Verification items for this drawing (mm, ordinates from the low corner). A direction names the side the tool comes from. Round coordinates to 2 decimals unless told otherwise and drop trailing zeros. Loops run counter-clockwise (first coordinate to the right, second up) from the corner with the lowest first, then second, coordinate; pieces in that order, holes last. Notation, with made-up numbers: (88, -15.5) - (125, -15.5) arc R27 cw to (125, 18.5) - close; hole circle Ø1 at (-23, -28). An arc over 180 degrees is marked (long way). Put each result on its own line as item: value.
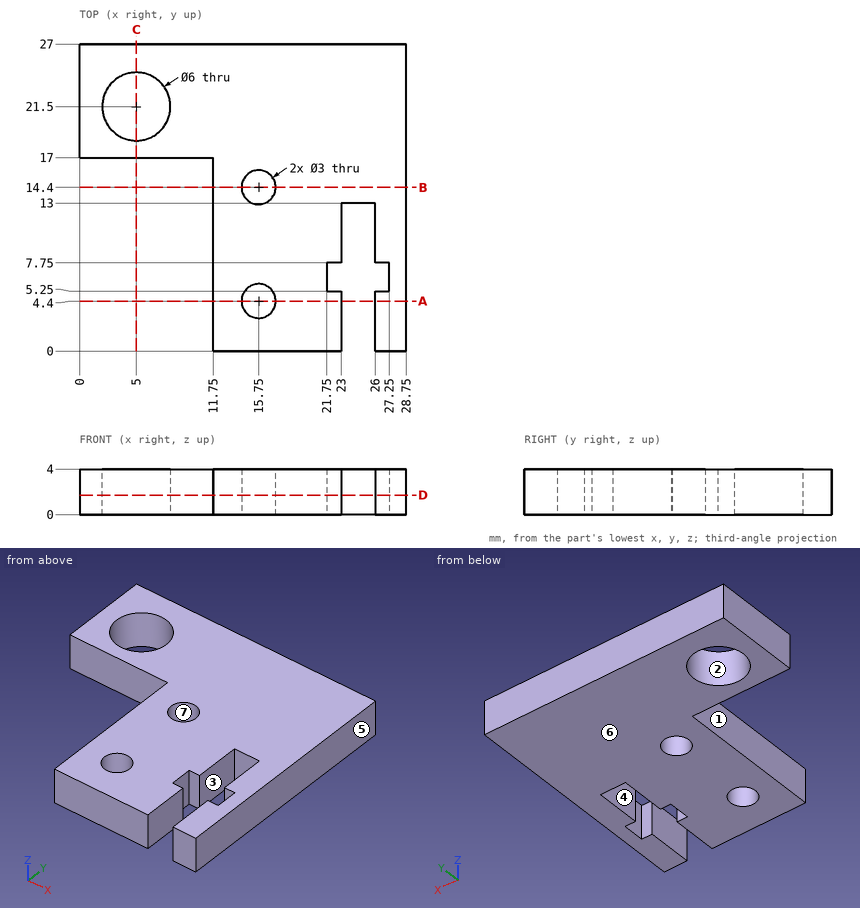
Item 1: Thickness scan on line 1 (Y direction, x = 15.75, z = 1.25); line 2 (X direction, y = 6.25, z = 3.8); line 3 (Y direction, x = 5, z = 1.95). Record the ranges inside material, lowest first. Write a range as from..to.
Filled sheet:
line 1: 0..2.9, 5.9..12.9, 15.9..27
line 2: 11.75..21.75, 27.25..28.75
line 3: 17..18.5, 24.5..27
Item 2: Go/stop test with flat-tipped pins: pin 1 (0.9 mm diameter, centred on x = 24.5, z = 1.5, fed in from -Y); pin 2 (1.2 mm diameter, centred on y = 11, z = 1.5, fed in from -X); pin 3 (1.2 mm diameter, centred on x = 7, z = 2, fed in from -Y). Record where each tip stops, or that it passes through.
Filled sheet:
pin 1: y = 13
pin 2: x = 11.75
pin 3: y = 17
Item 3: Section check D-D on z = 1.7. Enter the section's corners in (x, y), then the cut area to 3 significant figures.
Filled sheet:
outline: (0, 17) - (11.75, 17) - (11.75, 0) - (23, 0) - (23, 5.25) - (21.75, 5.25) - (21.75, 7.75) - (23, 7.75) - (23, 13) - (26, 13) - (26, 7.75) - (27.25, 7.75) - (27.25, 5.25) - (26, 5.25) - (26, 0) - (28.75, 0) - (28.75, 27) - (0, 27) - close; hole circle Ø6 at (5, 21.5); hole circle Ø3 at (15.75, 4.4); hole circle Ø3 at (15.75, 14.4)
area: 489 mm²
Item 4: Tool access check on the marked faces 1, 2 and 3. Record the directions out of +Z, -Z, +X, -X, +Y, -Y that give a thin tool (end or side, any length) a straight path to the whole face; none if there is none.
Filled sheet:
face 1: +Z, -Z, -X, -Y
face 2: +Z, -Z
face 3: +Z, -Z, -Y
Item 5: Section check C-C on x = 5. Enter the section's corners in (y, z), then the cut area to 3 significant figures.
Filled sheet:
outline: (17, 0) - (18.5, 0) - (18.5, 4) - (17, 4) - close; (24.5, 0) - (27, 0) - (27, 4) - (24.5, 4) - close
area: 16.0 mm²
Item 6: Release check for a two-part mould opening along X. For the marked faces 4, 5, 6 and 7 record: +X half, -X half, draft (parallel to the pull), parting line (faces both ways), or undercut.
Filled sheet:
face 4: undercut
face 5: +X half
face 6: draft
face 7: undercut
Item 7: Section check B-B on y = 14.4. Enter the section's corners in (x, z).
Filled sheet:
outline: (11.75, 0) - (14.25, 0) - (14.25, 4) - (11.75, 4) - close; (17.25, 0) - (28.75, 0) - (28.75, 4) - (17.25, 4) - close
Item 8: Section check A-A on y = 4.4. Enter the section's corners in (x, z).
Filled sheet:
outline: (11.75, 0) - (14.25, 0) - (14.25, 4) - (11.75, 4) - close; (17.25, 0) - (23, 0) - (23, 4) - (17.25, 4) - close; (26, 0) - (28.75, 0) - (28.75, 4) - (26, 4) - close
